Input: part model. Units: mm. Frame: model coordinates. Face numbers are marked on the shaded views. A direction names the side the tool comes from. Round coordinates to 2 decimals unless told otherwise and drop trailing zeros. Loops run counter-clockwise (first coordinate to the right, second up) from the corner with the lowest first, then second, coordinate; pieces in that order, holes last. Notation, with made-up numbers: (85.5, 48.5) -> (95.5, 48.5) arc R19 ccw to (95.5, 57.5) -> close; hole circle Ø3 at (-36.75, -28). An arc over 180 degrees is marked (long way). One line per question, with ' | ' between items. Start each with the question number.
Q1. Material intervals for L1, parallel to Y at x = -8, z = 0.3; L2, parallel to X at y = -10, z = 0.55; L3, parallel to Z at x = 2.75, y = 3.75, sorted ascending.
Q2. Contact query for flat-ended pins moving along their axis: P1, Ø2.5, axis at x = 0, y = 10, coming from the -Z side; P2, Ø1.5, axis at x = -7.5, y = 10, coming from the +Z side; P3, Ø6, axis at y = 1.5, z = 11, coming from the -X side; P4, Ø3, axis at y = 2, z = 4.5, coming from the +X side. Output: stop coordinate, or through.
Q3. Cut plane A-A on y = 0. Return loops of the section in (x, z).
Q4. Cut plane B-B on x = -5.25. Return loops of the section in (y, z), and give its area (3 significant figures).
Q5. Access query for the marked faces 4 and 5. Directions: +Z, -Z, +X, -X, +Y, -Y. A direction counts if a zero-diameter tool reaches every point of the face in a straight line with its end or side. Return the directions, or none.
Q6. Mould query, pull axis Y, two halves, no side actions, for the marked faces 1, 2 and 3. Classes: pulls with the +Y half, pulls with the -Y half, needs draft (parallel to the pull), parting line crosses it, or undercut.
Q7. Cut plane C-C on y = 5.25. Return loops of the section in (x, z).
Q8. Cut plane D-D on x = 0.5. Return loops of the section in (y, z).
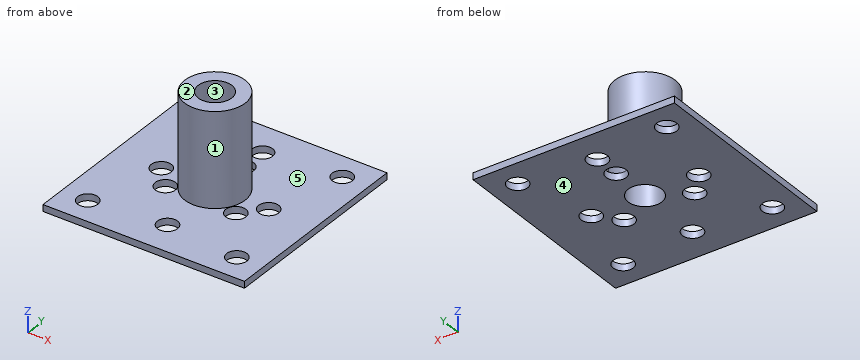
from build123d import *

# Parameters (mm, degrees)
SKETCH2_R           = 4.5
SKETCH2_R_2         = 2.5
BOSS_EXTRUDE4_DEPTH = 15
SKETCH3_W           = 30
SKETCH3_H           = 30
BOSS_EXTRUDE5_DEPTH = 1
SKETCH6_R           = 1.5
SKETCH6_R_2         = 2.5
CUT_EXTRUDE4_DEPTH  = 20


with BuildPart() as part:
    # Sketch2 → Boss-Extrude4 (new body)
    with BuildSketch(Plane.XY):
        Circle(SKETCH2_R)
        Circle(SKETCH2_R_2, mode=Mode.SUBTRACT)
    extrude(amount=BOSS_EXTRUDE4_DEPTH)

    # Sketch3 → Boss-Extrude5 (add)
    with BuildSketch(Plane.XY):
        Rectangle(SKETCH3_W, SKETCH3_H)
    extrude(amount=BOSS_EXTRUDE5_DEPTH)

    # Sketch6 → Cut-Extrude4 (cut)
    with BuildSketch(Plane.XY):
        with Locations((-11.101576465, -11.101576465)):
            Circle(SKETCH6_R)
        with Locations(Location((11.101576465, -11.101576465, 0), (0, 0, 180))):
            Circle(SKETCH6_R)
        with Locations((11.101576465, 11.101576465)):
            Circle(SKETCH6_R)
        with Locations(Location((-11.101576465, 11.101576465, 0), (0, 0, 180))):
            Circle(SKETCH6_R)
        with Locations((0, -10)):
            Circle(SKETCH6_R)
        with Locations(Location((0, 10, 0), (0, 0, 180))):
            Circle(SKETCH6_R)
        with Locations((-8, 0)):
            Circle(SKETCH6_R)
        with Locations(Location((8, 0, 0), (0, 0, 180))):
            Circle(SKETCH6_R)
        with Locations((0, 6.062177826)):
            Circle(SKETCH6_R)
        with Locations((5.25, -3.031088913)):
            Circle(SKETCH6_R)
        with Locations((-5.25, -3.031088913)):
            Circle(SKETCH6_R)
        Circle(SKETCH6_R_2)
    extrude(amount=CUT_EXTRUDE4_DEPTH, mode=Mode.SUBTRACT)


solid = part.part
Results:
1) L1: -15 to -1.5, 1.5 to 15 | L2: -15 to -12.12, -10.08 to -1.5, 1.5 to 10.08, 12.12 to 15 | L3: 0 to 1
2) P1: through | P2: z = 1 | P3: x = -4.5 | P4: x = 4.47
3) outline: (-15, 0) -> (-9.5, 0) -> (-9.5, 1) -> (-15, 1) -> close; (-6.5, 0) -> (-2.5, 0) -> (-2.5, 15) -> (-4.5, 15) -> (-4.5, 1) -> (-6.5, 1) -> close; (2.5, 0) -> (6.5, 0) -> (6.5, 1) -> (4.5, 1) -> (4.5, 15) -> (2.5, 15) -> close; (9.5, 0) -> (15, 0) -> (15, 1) -> (9.5, 1) -> close
4) outline: (-15, 0) -> (-4.53, 0) -> (-4.53, 1) -> (-15, 1) -> close; (-1.53, 0) -> (15, 0) -> (15, 1) -> (-1.53, 1) -> close | area: 27.0 mm^2
5) face 4: -Z, +X, -X, +Y, -Y | face 5: +Z
6) face 1: parting line crosses it | face 2: needs draft | face 3: undercut
7) outline: (-15, 0) -> (-1.26, 0) -> (-1.26, 1) -> (-15, 1) -> close; (1.26, 0) -> (15, 0) -> (15, 1) -> (1.26, 1) -> close
8) outline: (-15, 0) -> (-11.41, 0) -> (-11.41, 1) -> (-15, 1) -> close; (-8.59, 0) -> (-2.45, 0) -> (-2.45, 15) -> (-4.47, 15) -> (-4.47, 1) -> (-8.59, 1) -> close; (2.45, 0) -> (4.65, 0) -> (4.65, 1) -> (4.47, 1) -> (4.47, 15) -> (2.45, 15) -> close; (7.48, 0) -> (8.59, 0) -> (8.59, 1) -> (7.48, 1) -> close; (11.41, 0) -> (15, 0) -> (15, 1) -> (11.41, 1) -> close
